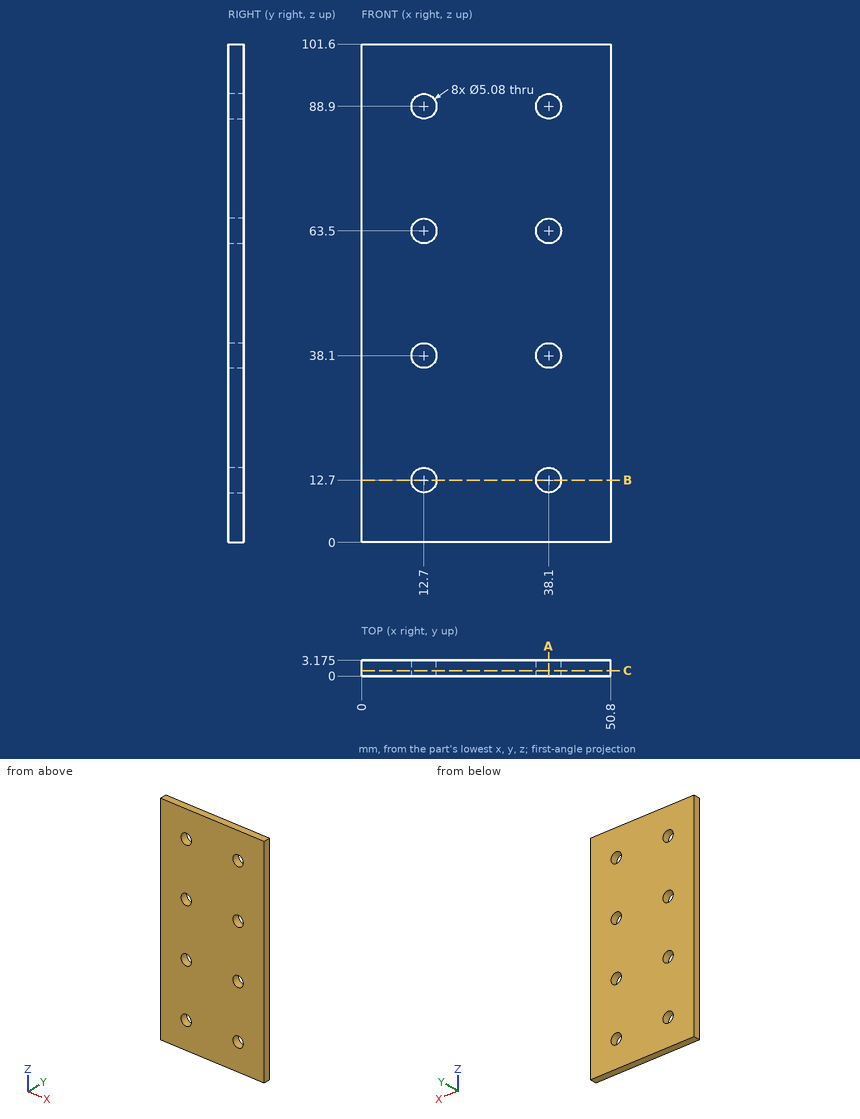
Answer from the drawing. Dimensions are ordinates in mm from the lowest x, y and z of the part. Give positions to 0.01 mm unless a question says otherwise; leave off trailing zeros. Loops run counter-clockwise (first coordinate to the right, second up) from the corner with the lowest first, then second, coordinate; pieces in that order, holes last. Notation, with made-up numbers: (54.5, 25) - (70.5, 25) arc R18 cw to (70.5, 55) - close; hole circle Ø6 at (42.5, -37). An arc over 180 degrees is marked (long way). Answer as CSV lines item,"result". Start each with the question number.
Item 1: A cutting plane is placed at B-B on z = 12.7. Determine the outline of the cut face in (x, y) (3 decimals).
Item 2: Find the intervals of material crossed by line 1 (X direction, y = 0.7, z = 63.5); line 2 (X direction, y = 2.05, z = 40); line 3 (Z direction, x = 11, y = 2.55), in increasing order. Write a range as from..to.
Item 3: This flat-tipped pin is pushed along its axis until it touches: pin 1 (1.5 mm diameter, centred on x = 38.5, y = 2.5, fed in from -Z). Where does it stop, or does it pass through?
Item 4: A cutting plane is placed at C-C on y = 1.1. Count the separate pieces of the cut face and the enclosed holes in it, then the cut area to 3 significant figures.
Item 5: A cutting plane is placed at A-A on x = 38.1. Determine the outline of the cut face in (y, z) (3 decimals), then the cut area to 3 significant figures.
Found:
1,outline,"(0, 0) - (10.16, 0) - (10.16, 3.175) - (0, 3.175) - close; (15.24, 0) - (35.56, 0) - (35.56, 3.175) - (15.24, 3.175) - close; (40.64, 0) - (50.8, 0) - (50.8, 3.175) - (40.64, 3.175) - close"
2,line 1,"x = 0..10.16, 15.24..35.56, 40.64..50.8"
2,line 2,"x = 0..11.01, 14.39..36.41, 39.79..50.8"
2,line 3,"z = 0..10.81, 14.59..36.21, 39.99..61.61, 65.39..87.01, 90.79..101.6"
3,pin 1,"stops at z = 0"
4,separate pieces,"1"
4,enclosed holes,"8"
4,area,"5,000 mm^2"
5,outline,"(0, 0) - (3.175, 0) - (3.175, 10.16) - (0, 10.16) - close; (0, 15.24) - (3.175, 15.24) - (3.175, 35.56) - (0, 35.56) - close; (0, 40.64) - (3.175, 40.64) - (3.175, 60.96) - (0, 60.96) - close; (0, 66.04) - (3.175, 66.04) - (3.175, 86.36) - (0, 86.36) - close; (0, 91.44) - (3.175, 91.44) - (3.175, 101.6) - (0, 101.6) - close"
5,area,"258 mm^2"
